Work out the finished part from the listing and answer in its coordinate system (mm). Round coordinates to 2 decimals unless told otherwise and drop trailing zeros. Loops run counter-clockwise (first coordinate to the right, second up) from the corner with the lowest first, then second, coordinate; pieces in that order, holes last. Notation, with made-up numbers: (24, 15.5) -> (36, 15.5) arc R19 cw to (36, 41.5) -> close; hole circle Ø3 at (-26, 27). An arc over 180 degrees is marked (long way). Write item = value, one per line. Start each with the question number.
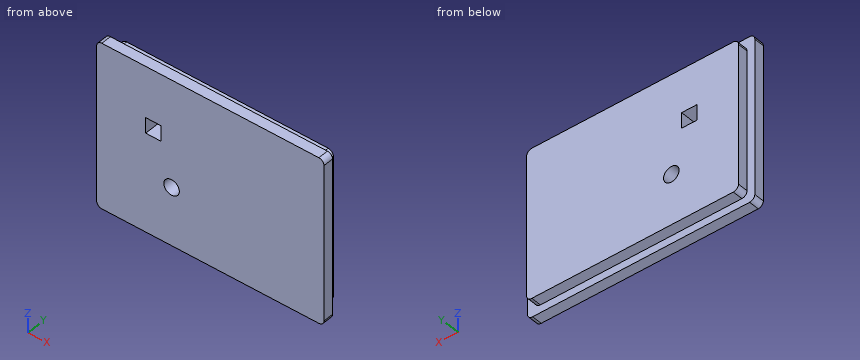
Autodesk Fusion 360 part; units mm, degrees
sketch "Sketch1" plane through (0, 0, 0) normal (0, 1, 0) x (1, 0, 0) in component "Lid"
sketch "Sketch2" plane through (0, 0, 0) normal (0, 1, 0) x (1, 0, 0) in component "Lid"
sketch "Sketch3" plane through (0, 0, 0) normal (0, 1, 0) x (1, 0, 0) in component "Lid"
  line L0 (55.88, 40.64) -> (-55.88, 40.64)
  line L1 (-55.88, 40.64) -> (-55.88, -40.64)
  line L2 (-55.88, -40.64) -> (55.88, -40.64)
  line L3 (55.88, -40.64) -> (55.88, 40.64)
  line L4 (55.88, 40.64) -> (-55.88, -40.64) construction
  line L5 (-55.88, 40.64) -> (55.88, -40.64) construction
  dimension "d1" = 111.76
  dimension "d2" = 81.28
extrude "Extrude1" add sketch "Sketch3" along normal blind 5.08 in component "Lid"
sketch "Sketch4" plane through (0, 5.08, 0) normal (0, 1, 0) x (-1, 0, 0) in component "Lid"
  line L0 (-55.88, 40.64) -> (-55.88, -40.64)
  line L1 (-55.88, -40.64) -> (55.88, -40.64)
  line L2 (55.88, -40.64) -> (55.88, 40.64)
  line L3 (55.88, 40.64) -> (-55.88, 40.64)
  line L4 (-52.07, -36.83) -> (52.07, -36.83)
  line L5 (52.07, -36.83) -> (52.07, 36.83)
  line L6 (52.07, 36.83) -> (-52.07, 36.83)
  line L7 (-52.07, 36.83) -> (-52.07, -36.83)
  line L8 (-52.07, -36.83) -> (52.07, 36.83) construction
  line L9 (52.07, -36.83) -> (-52.07, 36.83) construction
  dimension "d5" = 104.14
  dimension "d6" = 73.66
extrude "Extrude2" add sketch "Sketch4" along normal blind 5.08 contours L4 L5 L6 L7 in component "Lid"
fillet "Fillet1" radius 2.54 8 edges at (52.07, 7.62, 36.83) (-52.07, 7.62, 36.83) (52.07, 7.62, -36.83) (-52.07, 7.62, -36.83) (-55.88, 2.54, -40.64) (55.88, 2.54, -40.64) (55.88, 2.54, 40.64) (-55.88, 2.54, 40.64) in component "Lid"
sketch "Sketch1 (2)" plane through (0, 0, 0) normal (0, -1, 0) x (1, 0, 0)
  arc A0 (-53.34, 40.64) -> (-55.88, 38.1) centre (-53.34, 38.1) ccw
  line L0 (-55.88, 38.1) -> (-55.88, -38.1)
  arc A1 (-55.88, -38.1) -> (-53.34, -40.64) centre (-53.34, -38.1) ccw
  line L1 (-53.34, -40.64) -> (53.34, -40.64)
  arc A2 (53.34, -40.64) -> (55.88, -38.1) centre (53.34, -38.1) ccw
  line L2 (55.88, -38.1) -> (55.88, 38.1)
  arc A3 (55.88, 38.1) -> (53.34, 40.64) centre (53.34, 38.1) ccw
  line L3 (53.34, 40.64) -> (-53.34, 40.64)
  line L4 (43.815, 27.94) -> (-43.815, 27.94)
  line L5 (-43.815, 27.94) -> (-43.815, -27.94)
  line L6 (-43.815, -27.94) -> (43.815, -27.94)
  line L7 (43.815, -27.94) -> (43.815, 27.94)
  line L8 (43.815, 27.94) -> (-43.815, -27.94) construction
  line L9 (-43.815, 27.94) -> (43.815, -27.94) construction
  dimension "d10" = 87.63
  dimension "d11" = 55.88
sketch "Sketch2 (2)" plane through (0, 0, 0) normal (0, -1, 0) x (1, 0, 0)
  circle A0 centre (-19.05, -12.065) radius 3.81
  dimension "d12" = 7.62
  dimension "d13" = 24.765
  dimension "d14" = 15.875
extrude "Extrude3" cut sketch "Sketch2 (2)" against normal blind 10.16 in component "Lid"
sketch "Sketch3 (2)" plane through (0, 0, 0) normal (0, 1, 0) x (1, 0, 0)
  line L0 (-24.13, -15.494) -> (-31.75, -15.494)
  line L1 (-31.75, -15.494) -> (-31.75, -7.874)
  line L2 (-31.75, -7.874) -> (-24.13, -7.874)
  line L3 (-24.13, -7.874) -> (-24.13, -15.494)
  line L4 (-24.13, -15.494) -> (-31.75, -7.874) construction
  line L5 (-31.75, -15.494) -> (-24.13, -7.874) construction
  dimension "d17" = 7.62
  dimension "d18" = 7.62
  dimension "d19" = 39.624
  dimension "d20" = 15.875
extrude "Extrude4" cut sketch "Sketch3 (2)" along normal blind 10.16 in component "Lid"
component "Lid" placed x (1, 0, 0) y (0, 1, 0) z (0, 0, 1) at (0, 0, 0)
Item 1: Section A-A (x = -19.05) is taken. Determine the outline of the cut face in (y, z) (3 decimals).
Item 2: Section D-D (y = 7.75) is taken. Determine the outline of the cut face in (x, z) (3 decimals), then the cut area to 3 significant figures.
Item 3: Section B-B (z = 13) is taken. Determine the outline of the cut face in (x, y).
Item 4: Section C-C (x = -38) is taken. Determine the outline of the cut face in (y, z).
Item 5: Flat-ended cylindrical pins translate along their axes: pin 1 (1.5 mm diameter, centred on x = -20.5, y = 8, fed in from +Z); pin 2 (4 mm diameter, centred on y = 8, z = 6, fed in from -X); pin 3 (2.5 mm diameter, centred on y = 8.5, z = -7.5, fed in from +X). Find the tip coordinate at first contact, or state that the pin passes through.
Item 6: Find the intervals of material crossed by line 1 along Z through (x, y) = (-19.05, 4.25) (3 decimals); line 2 along Z through (x, y) = (-19.05, 6.25) (3 decimals); line 3 along Z through (x, y) = (10, 9.5), in increasing order. Write a range as [from, to].
Worked answers:
q1.outline = (0, -40.64) -> (5.08, -40.64) -> (5.08, -36.83) -> (10.16, -36.83) -> (10.16, -15.875) -> (0, -15.875) -> close; (0, -8.255) -> (10.16, -8.255) -> (10.16, 36.83) -> (5.08, 36.83) -> (5.08, 40.64) -> (0, 40.64) -> close
q2.outline = (-52.07, -34.29) arc R2.54 ccw to (-49.53, -36.83) -> (49.53, -36.83) arc R2.54 ccw to (52.07, -34.29) -> (52.07, 34.29) arc R2.54 ccw to (49.53, 36.83) -> (-49.53, 36.83) arc R2.54 ccw to (-52.07, 34.29) -> close; hole (-31.75, 7.874) -> (-24.13, 7.874) -> (-24.13, 15.494) -> (-31.75, 15.494) -> close; hole circle Ø7.62 at (-19.05, -12.065)
q2.area = 7,560 mm2
q3.outline = (-55.88, 0) -> (-31.75, 0) -> (-31.75, 10.16) -> (-52.07, 10.16) -> (-52.07, 5.08) -> (-55.88, 5.08) -> close; (-24.13, 0) -> (55.88, 0) -> (55.88, 5.08) -> (52.07, 5.08) -> (52.07, 10.16) -> (-24.13, 10.16) -> close
q4.outline = (0, -40.64) -> (5.08, -40.64) -> (5.08, -36.83) -> (10.16, -36.83) -> (10.16, 36.83) -> (5.08, 36.83) -> (5.08, 40.64) -> (0, 40.64) -> close
q5.pin_1 = 36.83
q5.pin_2 = -52.07
q5.pin_3 = 52.07
q6.line_1 = [-40.64, -15.875], [-8.255, 40.64]
q6.line_2 = [-36.83, -15.875], [-8.255, 36.83]
q6.line_3 = [-36.83, 36.83]
